```python
from build123d import *

# Parameters (mm, degrees)
Y_KSEKLIK_EKSTR_ZYON1_DEPTH = 2
KES_EKSTR_ZYON1_DEPTH       = 1
IZIM6_R                     = 1.501031458
IZIM6_R_2                   = 1.001031998
IZIM6_R_3                   = 1.5
IZIM6_R_4                   = 1.00000054
Y_KSEKLIK_EKSTR_ZYON3_DEPTH = 3.425399462


with BuildPart() as part:
    # Çizim1 → Yükseklik-Ekstrüzyon1 (new body)
    with BuildSketch(Plane(origin=(0, 0, 0), x_dir=(1, 0, 0), z_dir=(0, 1, 0))):
        with BuildLine():
            Line((69.354296896, 0), (22.205894341, 0))
            ThreePointArc((22.205894341, 0), (20.084057526, 0.878893586), (19.20516394, 3.000730401))
            Line((19.20516394, 3.000730401), (19.20516394, 28.999269019))
            ThreePointArc((19.20516394, 28.999269019), (20.084057735, 31.121106339), (22.205895054, 32.000000134))
            Line((22.205895054, 32.000000134), (69.204054025, 31.999999983))
            ThreePointArc((69.204054025, 31.999999983), (72.103447224, 30.757719929), (73.203992826, 27.80161776))
            Line((73.203992826, 27.80161776), (73.205163894, 3.84969587))
            ThreePointArc((73.205163894, 3.84969587), (72.076857039, 1.127478795), (69.354296896, 0))
        make_face()
    extrude(amount=Y_KSEKLIK_EKSTR_ZYON1_DEPTH)

    # Çizim2 → Kes-Ekstrüzyon1 (cut)
    with BuildSketch(Plane.XZ):
        with BuildLine():
            Line((22.205894341, 0), (69.354296896, 0))
            ThreePointArc((69.354296896, 0), (72.076886077, -1.127507843), (73.205163905, -3.849778017))
            Line((73.205163905, -3.849778017), (73.204578669, -27.814116173))
            ThreePointArc((73.204578669, -27.814116173), (72.09912832, -30.762246017), (69.204054025, -31.999999983))
            Line((69.204054025, -31.999999983), (22.205895054, -32.000000134))
            ThreePointArc((22.205895054, -32.000000134), (20.084057735, -31.121106339), (19.20516394, -28.999269019))
            Line((19.20516394, -28.999269019), (19.20516394, -3.000730401))
            ThreePointArc((19.20516394, -3.000730401), (20.084057526, -0.878893586), (22.205894341, 0))
        make_face()
        with BuildLine():
            Line((22.205894341, -0.5), (69.354296896, -0.5))
            ThreePointArc((69.354296896, -0.5), (71.723357422, -1.481085951), (72.705163917, -3.849847954))
            Line((72.705163917, -3.849847954), (72.704578383, -27.82580896))
            ThreePointArc((72.704578383, -27.82580896), (71.741441976, -30.412825453), (69.204054025, -31.499999983))
            Line((69.204054025, -31.499999983), (22.205895054, -31.500000134))
            ThreePointArc((22.205895054, -31.500000134), (20.437611125, -30.767552948), (19.70516394, -28.999269019))
            Line((19.70516394, -28.999269019), (19.70516394, -3.000730401))
            ThreePointArc((19.70516394, -3.000730401), (20.437610916, -1.232446977), (22.205894341, -0.5))
        make_face(mode=Mode.SUBTRACT)
    extrude(amount=-KES_EKSTR_ZYON1_DEPTH, mode=Mode.SUBTRACT)

    # Çizim6 → Yükseklik-Ekstrüzyon3 (add)
    # profile 1 of 2: a face of its own
    with BuildSketch(Plane.XZ):
        with Locations(Location((22.205894341, -3.000730401, 0), (0, 0, 90))):
            Circle(IZIM6_R)
        with Locations(Location((22.205894341, -3.000730401, 0), (0, 0, 90))):
            Circle(IZIM6_R_2, mode=Mode.SUBTRACT)
    # profile 2 of 2: a face of its own
    with BuildSketch(Plane.XZ):
        with Locations(Location((69.70516394, -25.900001, 0), (0, 0, 90))):
            Circle(IZIM6_R_3)
        with Locations((69.70516394, -25.900001)):
            Circle(IZIM6_R_4, mode=Mode.SUBTRACT)
    extrude(amount=Y_KSEKLIK_EKSTR_ZYON3_DEPTH)


solid = part.part
```
For this review, take the finished solid that the model builds, in its own axes (mm). A direction names the side the tool comes from. Give positions to 0.01 mm unless a question says otherwise; leave off trailing zeros. Write each loop counter-clockwise with the first axis right and the second up, starting at its lowest first coordinate (ties: lowest second). Pieces come first, ordered by that corner, then holes. Notation, with made-up numbers: M -17.5,77 L 27.5,77 A22 cw 27.5,89 Z; hole C 71.5,18 d9. An arc over 180 degrees is marked long. One line per item, written item: value.
1) For line 1 (X direction, y = -2.65, z = -3); line 2 (Y direction, x = 36, z = -2.5); line 3 (Z direction, x = 35, y = 0.95), list the stretches that pass through material, from the lowest coordinate up. Write a range as from..to.
Results are:
line 1: x = 20.7..21.2, 23.21..23.71
line 2: y = 0..2
line 3: z = -31.5..-0.5
2) Take a section at C-C, the plane y = -0.6. Write out the cut boundary in (x, z), then the cut area to 3 significant figures.
Results are:
outline: C 22.21,-3 d3; C 69.71,-25.9 d3; hole C 22.21,-3 d2; hole C 69.71,-25.9 d2
area: 7.86 mm²
3) For P1, Ø0.6, axis at x = 69.5, z = -26, coming from the -Y side; P2, Ø0.8, axis at y = 0.5, z = -18, coming from the +X side; P3, Ø1.5, axis at y = -2.5, z = -12.5, coming from the -X side; P4, Ø1.1, axis at y = 1.5, z = -16, coming from the +X side, all flat-tipped, find the tip position at first contact; note any pin that passes through.
Results are:
P1: stops at y = 0
P2: stops at x = 72.7
P3: passes through
P4: stops at x = 73.2
4) For faces 4 (the flat face through (46, 0.5, -31.5)), 5 (the flat face through (70, 0, -26)), 6 (the cylindrical face through (20.46, 0.49, -30.79)), 7 (the flat face through (19.705, 0.5, -16.2)), list the 3-axis set-ups (+Z, -Z, +X, -X, +Y, -Y) from which the entire face can be reached by the end or side of a thin tool; tool diameter is ignored.
Results are:
face 4: -Z, +X, -X, -Y
face 5: -Y
face 6: -Z, -X, -Y
face 7: +Z, -Z, -X, -Y
5) Take a section at A-A, the plane x = 26.5. Write out the cut boundary in (y, z).
Results are:
outline: M 0,-31.5 L 1,-31.5 L 1,-32 L 2,-32 L 2,0 L 1,0 L 1,-0.5 L 0,-0.5 Z
6) The part is to be moulded in two halves that separate along X. For faces 1 (the flat face through (46.1, 1.5, 0)), 2 (the cylindrical face through (72.11, 1.49, -1.16)), 3 (the cylindrical face through (21.362, -1.689, -2.463)), say which applies: +X half, -X half, draft (parallel to the pull), parting line (faces both ways), or undercut.
Results are:
face 1: draft
face 2: +X half
face 3: undercut
7) Take a section at B-B, the plane z = -9. Write out the cut boundary in (x, y), then the cut area to 3 significant figures.
Results are:
outline: M 19.21,1 L 19.71,1 L 19.71,0 L 72.71,0 L 72.71,1 L 73.2,1 L 73.2,2 L 19.21,2 Z
area: 107 mm²
